For this review, take the finished solid that the model builds, in its own axes (mm). A direction names the side the tool comes from. Give positions to 0.01 mm unless a question says otherwise; leave off trailing zeros. Loops run counter-clockwise (first coordinate to the right, second up) from the corner with the lowest first, then second, coordinate; pieces in that order, holes last. Notation, with made-up numbers: (-7, -22) - (-3, -22) arc R14 ccw to (-3, 3) - close; hole circle Ø9 at (57, 48.5). An arc over 180 degrees is marked (long way). Put each result on its own line as item: value.
from build123d import *

# Parameters (mm, degrees)
SKETCH_1_W                   = 60
SKETCH_1_H                   = 40
SKETCH_1_W_2                 = 56
SKETCH_1_H_2                 = 36
EXTRUDE_1_DEPTH              = 299
HOLE_WIZARD_M31_AT_2_COUNT   = 2
HOLE_WIZARD_M31_AT_2_PITCH   = 22
HOLE_WIZARD_M32_AT_2_COUNT   = 2
HOLE_WIZARD_M32_AT_2_PITCH   = 22
HOLE_WIZARD_M33_AT_2_COUNT   = 2
HOLE_WIZARD_M33_AT_2_PITCH   = 16
HOLE_WIZARD_M34_AT_2_COUNT   = 2
HOLE_WIZARD_M34_AT_2_PITCH   = 16
CUT_EXTRUDE_4347_REACH       = 42
SKETCH_12_R                  = 4
CUT_EXTRUDE_3_REACH          = 62
SKETCH_15_R                  = 4
SKETCH_15_R_2                = 4.5
HOLE_WIZARD_4_401_AT_2_COUNT = 2
HOLE_WIZARD_4_401_AT_2_PITCH = 12
HOLE_WIZARD_4_401_AT_3_COUNT = 2
HOLE_WIZARD_4_401_AT_3_PITCH = 18.439088915
HOLE_WIZARD_4_401_AT_4_COUNT = 2
HOLE_WIZARD_4_401_AT_4_PITCH = 14


with BuildPart() as part:
    # Эскиз1 → Вытянуть1 (new body)
    with BuildSketch(Plane.XY):
        Rectangle(SKETCH_1_W, SKETCH_1_H)
        Rectangle(SKETCH_1_W_2, SKETCH_1_H_2, mode=Mode.SUBTRACT)
    extrude(amount=EXTRUDE_1_DEPTH)

    # Эскиз2 → Hole Wizard M31 (revolve, cut)
    with BuildSketch(Plane(origin=(-30, 11, 292), x_dir=(0, 0, 1), z_dir=(0, 1, 0))):
        Polygon((0, 0), (0, 2), (1.85, 2), (1.6, 1.75), (1.6, 0.25), (1.85, 0), align=None)
    hole_wizard_m31 = revolve(axis=Axis((-36.35, 11, 292), (1, 0, 0)), mode=Mode.SUBTRACT)

    # Hole Wizard M31 at 2: Hole Wizard M31 ×2
    with Locations(*[(0, -i * HOLE_WIZARD_M31_AT_2_PITCH, 0) for i in range(1, HOLE_WIZARD_M31_AT_2_COUNT)]):
        add(hole_wizard_m31, mode=Mode.SUBTRACT)

    # Эскиз4 → Отверстие с зазором M32 (revolve, cut)
    with BuildSketch(Plane(origin=(30, -11, 292), x_dir=(0, 0, -1), z_dir=(0, 1, 0))):
        Polygon((0, 0), (0, 2), (1.85, 2), (1.6, 1.75), (1.6, 0.25), (1.85, 0), align=None)
    hole_wizard_m32 = revolve(axis=Axis((36.35, -11, 292), (-1, 0, 0)), mode=Mode.SUBTRACT)

    # Отверстие с зазором M32 at 2: Отверстие с зазором M32 ×2
    with Locations(*[(0, i * HOLE_WIZARD_M32_AT_2_PITCH, 0) for i in range(1, HOLE_WIZARD_M32_AT_2_COUNT)]):
        add(hole_wizard_m32, mode=Mode.SUBTRACT)

    # Эскиз6 → Отверстие с зазором M33 (revolve, cut)
    with BuildSketch(Plane(origin=(-8, -20, 290), x_dir=(0, 0, -1), z_dir=(1, 0, 0))):
        Polygon((0, 0), (0, 2), (1.85, 2), (1.6, 1.75), (1.6, 0.25), (1.85, 0), align=None)
    hole_wizard_m33 = revolve(axis=Axis((-8, -26.35, 290), (0, 1, 0)), mode=Mode.SUBTRACT)

    # Отверстие с зазором M33 at 2: Отверстие с зазором M33 ×2
    with Locations(*[(i * HOLE_WIZARD_M33_AT_2_PITCH, 0, 0) for i in range(1, HOLE_WIZARD_M33_AT_2_COUNT)]):
        add(hole_wizard_m33, mode=Mode.SUBTRACT)

    # Эскиз8 → Отверстие с зазором M34 (revolve, cut)
    with BuildSketch(Plane(origin=(8, 20, 290), x_dir=(0, 0, 1), z_dir=(1, 0, 0))):
        Polygon((0, 0), (0, 2), (1.85, 2), (1.6, 1.75), (1.6, 0.25), (1.85, 0), align=None)
    hole_wizard_m34 = revolve(axis=Axis((8, 26.35, 290), (0, -1, 0)), mode=Mode.SUBTRACT)

    # Отверстие с зазором M34 at 2: Отверстие с зазором M34 ×2
    with Locations(*[(-i * HOLE_WIZARD_M34_AT_2_PITCH, 0, 0) for i in range(1, HOLE_WIZARD_M34_AT_2_COUNT)]):
        add(hole_wizard_m34, mode=Mode.SUBTRACT)

    # Эскиз12 → Cut-Extrude 4347 (cut, up to next)
    with BuildSketch(Plane(origin=(0, -20, 0), x_dir=(1, 0, 0), z_dir=(0, 1, 0)), mode=Mode.PRIVATE) as cut_extrude_4347_sk1:
        with Locations((19, -240.5)):
            Circle(SKETCH_12_R)
    cut_extrude_4347_tool1 = extrude(cut_extrude_4347_sk1.sketch, amount=CUT_EXTRUDE_4347_REACH, mode=Mode.PRIVATE) & part.part
    add(cut_extrude_4347_tool1.solids().sort_by_distance((19, -20, 240.5))[0], mode=Mode.SUBTRACT)
    # Эскиз12 → Cut-Extrude 4347 (cut, up to next)
    with BuildSketch(Plane(origin=(0, -20, 0), x_dir=(1, 0, 0), z_dir=(0, 1, 0)), mode=Mode.PRIVATE) as cut_extrude_4347_sk2:
        with Locations((12, -35)):
            Circle(SKETCH_12_R)
    cut_extrude_4347_tool2 = extrude(cut_extrude_4347_sk2.sketch, amount=CUT_EXTRUDE_4347_REACH, mode=Mode.PRIVATE) & part.part
    add(cut_extrude_4347_tool2.solids().sort_by_distance((12, -20, 35))[0], mode=Mode.SUBTRACT)

    # Эскиз15 → Вырез-Вытянуть3 (cut, up to next)
    with BuildSketch(Plane(origin=(30, 0, 0), x_dir=(0, 0, -1), z_dir=(1, 0, 0)), mode=Mode.PRIVATE) as cut_extrude_3_sk1:
        with Locations((-37, 13)):
            Circle(SKETCH_15_R)
    cut_extrude_3_tool1 = extrude(cut_extrude_3_sk1.sketch, amount=-CUT_EXTRUDE_3_REACH, mode=Mode.PRIVATE) & part.part
    add(cut_extrude_3_tool1.solids().sort_by_distance((30, 13, 37))[0], mode=Mode.SUBTRACT)
    # Эскиз15 → Вырез-Вытянуть3 (cut, up to next)
    with BuildSketch(Plane(origin=(30, 0, 0), x_dir=(0, 0, -1), z_dir=(1, 0, 0)), mode=Mode.PRIVATE) as cut_extrude_3_sk2:
        with Locations((-268, 13)):
            Circle(SKETCH_15_R)
    cut_extrude_3_tool2 = extrude(cut_extrude_3_sk2.sketch, amount=-CUT_EXTRUDE_3_REACH, mode=Mode.PRIVATE) & part.part
    add(cut_extrude_3_tool2.solids().sort_by_distance((30, 13, 268))[0], mode=Mode.SUBTRACT)
    # Эскиз15 → Вырез-Вытянуть3 (cut, up to next)
    with BuildSketch(Plane(origin=(30, 0, 0), x_dir=(0, 0, -1), z_dir=(1, 0, 0)), mode=Mode.PRIVATE) as cut_extrude_3_sk3:
        with Locations((-228, 11.5)):
            Circle(SKETCH_15_R_2)
    cut_extrude_3_tool3 = extrude(cut_extrude_3_sk3.sketch, amount=-CUT_EXTRUDE_3_REACH, mode=Mode.PRIVATE) & part.part
    add(cut_extrude_3_tool3.solids().sort_by_distance((30, 11.5, 228))[0], mode=Mode.SUBTRACT)

    # Эскиз16 → Отверстие обработанное метчиком #4-401 (revolve, cut)
    with BuildSketch(Plane(origin=(30, 16.5, 235), x_dir=(0, 0, -1), z_dir=(0, 1, 0))):
        Polygon((0, 0), (0, 2), (1.524, 2), (1.1303, 1.724328292), (1.1303, 0.275671708), (1.524, 0), align=None)
    hole_wizard_4_401 = revolve(axis=Axis((36.35, 16.5, 235), (-1, 0, 0)), mode=Mode.SUBTRACT)

    # Отверстие обработанное метчиком #4-401 at 2: Отверстие обработанное метчиком #4-401 ×2
    with Locations(*[(0, -i * HOLE_WIZARD_4_401_AT_2_PITCH, 0) for i in range(1, HOLE_WIZARD_4_401_AT_2_COUNT)]):
        add(hole_wizard_4_401, mode=Mode.SUBTRACT)

    # Отверстие обработанное метчиком #4-401 at 3: Отверстие обработанное метчиком #4-401 ×2
    with Locations(*[Vector(0, -0.650791373, -0.759256602) * (i * HOLE_WIZARD_4_401_AT_3_PITCH) for i in range(1, HOLE_WIZARD_4_401_AT_3_COUNT)]):
        add(hole_wizard_4_401, mode=Mode.SUBTRACT)

    # Отверстие обработанное метчиком #4-401 at 4: Отверстие обработанное метчиком #4-401 ×2
    with Locations(*[(0, 0, -i * HOLE_WIZARD_4_401_AT_4_PITCH) for i in range(1, HOLE_WIZARD_4_401_AT_4_COUNT)]):
        add(hole_wizard_4_401, mode=Mode.SUBTRACT)


solid = part.part
1) Take a section at C-C on x = 19. State the section outline as (y, z) points, and give its area (3 significant figures).
Geometry check:
outline: (-20, 0) - (-18, 0) - (-18, 236.5) - (-20, 236.5) - close; (-20, 244.5) - (-18, 244.5) - (-18, 299) - (-20, 299) - close; (18, 0) - (20, 0) - (20, 299) - (18, 299) - close
area: 1,180 mm²
2) Wall thickness on line 1 (Y direction, x = 3, z = 120.5); line 2 (X direction, y = 4.5, z = 146); line 3 (X direction, y = -19, z = 290): over which ranges is each line inside the solid? List them lowest first.
Geometry check:
line 1: y = -20 to -18, 18 to 20
line 2: x = -30 to -28, 28 to 30
line 3: x = -30 to -9.6, -6.4 to 6.4, 9.6 to 30
3) Draft analysis for pull direction Y (two halves, no side actions). For faces 1 (the face through (0, 20, 147)), 2 (the face through (30, 0, 147)), 3 (the face through (-28, 0, 147)), state which applies: pulls with the +Y half, pulls with the -Y half, needs draft (parallel to the pull), parting line crosses it, or undercut.
Geometry check:
face 1: pulls with the +Y half
face 2: needs draft
face 3: undercut
4) Take a section at D-D on y = -1.5. State the section outline as (x, z) points, and give its area (3 significant figures).
Geometry check:
outline: (-30, 0) - (-28, 0) - (-28, 299) - (-30, 299) - close; (28, 0) - (30, 0) - (30, 299) - (28, 299) - close
area: 1,200 mm²
5) Take a section at B-B on z = 214. State the section outline as (x, y) points.
Geometry check:
outline: (-30, -20) - (30, -20) - (30, 20) - (-30, 20) - close; hole (-28, -18) - (28, -18) - (28, 18) - (-28, 18) - close
6) Take a section at A-A on x = -22.5. State the section outline as (y, z) points.
Geometry check:
outline: (-20, 0) - (-18, 0) - (-18, 299) - (-20, 299) - close; (18, 0) - (20, 0) - (20, 299) - (18, 299) - close
7) For faces 4 (the face through (29.01, 15.7, 39.95)), 5 (the face through (21.15, -19.014, 237.127)), 6 (the face through (0, -18, 147)), list the 3-axis set-ups (+Z, -Z, +X, -X, +Y, -Y) from which the entire face can be reached by the end or side of a thin tool; tool diameter is ignored.
Geometry check:
face 4: +X
face 5: -Y
face 6: +Z, -Z
8) Insertion check: pin 1 Ø3.5 at (y, z) = (11, 292) entering from -X; pin 2 Ø2.5 at (y, z) = (4.5, 235) entering from +X. Each pin has a flat end and moves straight along its axis. Give the tip position at first contact, or say it passes through.
Geometry check:
pin 1: stops at x = -29.9
pin 2: stops at x = 29.81
